```python
from build123d import *

# Parameters (mm, degrees)
SKETCH1_W           = 70
SKETCH1_H           = 70
BOSS_EXTRUDE1_DEPTH = 10
SKETCH2_R           = 30
SKETCH2_R_2         = 27.45
BOSS_EXTRUDE2_DEPTH = 5
FILLET1_R           = 2.5
BOSS_EXTRUDE3_DEPTH = 10
SKETCH5_R           = 1.5
SKETCH5_W           = 70
SKETCH5_H           = 10
BOSS_EXTRUDE5_DEPTH = 3


with BuildPart() as part:
    # Sketch1 → Boss-Extrude1 (new body)
    with BuildSketch(Plane.XY):
        Rectangle(SKETCH1_W, SKETCH1_H)
    extrude(amount=BOSS_EXTRUDE1_DEPTH)

    # Sketch2 → Boss-Extrude2 (add)
    with BuildSketch(Plane.XY.offset(10)):
        Circle(SKETCH2_R)
        Circle(SKETCH2_R_2, mode=Mode.SUBTRACT)
    extrude(amount=BOSS_EXTRUDE2_DEPTH)

    # Fillet1
    fillet1_edges = [part.edges().sort_by_distance(p)[0] for p in [
        (-35, 35, 5),
        (35, 35, 5),
    ]]
    fillet(fillet1_edges, radius=FILLET1_R)

    # Sketch3 → Boss-Extrude3 (add)
    with BuildSketch(Plane(origin=(0, 0, 0), x_dir=(-1, 0, 0), z_dir=(0, 0, -1))):
        Polygon((-20.75, -38.5), (-15.75, -38.5), (-15.75, -41.5), (-30.75, -41.5), (-30.75, -38.5), (-25.75, -38.5), (-25.75, -35), (-20.75, -35), align=None)
        Polygon((30.75, -38.5), (30.75, -41.5), (15.75, -41.5), (15.75, -38.5), (20.75, -38.5), (20.75, -35), (25.75, -35), (25.75, -38.5), align=None)
    extrude(amount=-BOSS_EXTRUDE3_DEPTH)

    # Sketch5 → Boss-Extrude5 (add)
    with BuildSketch(Plane.XZ.offset(35)):
        with BuildLine():
            Line((5, -5), (35, -5))
            ThreePointArc((35, -5), (38.535533906, -3.535533906), (40, 0))
            Line((40, 0), (40, 10))
            ThreePointArc((40, 10), (38.535533906, 13.535533906), (35, 15))
            Line((35, 15), (-35, 15))
            ThreePointArc((-35, 15), (-38.535533906, 13.535533906), (-40, 10))
            Line((-40, 10), (-40, 0))
            ThreePointArc((-40, 0), (-38.535533906, -3.535533906), (-35, -5))
            Line((-35, -5), (-5, -5))
            Line((-5, -5), (-5, -5.5))
            ThreePointArc((-5, -5.5), (-4.853553391, -5.853553391), (-4.5, -6))
            Line((-4.5, -6), (4.5, -6))
            ThreePointArc((4.5, -6), (4.853553391, -5.853553391), (5, -5.5))
            Line((5, -5.5), (5, -5))
        make_face()
        with Locations(Location((0, -3, 0), (0, 0, 270))):
            Circle(SKETCH5_R, mode=Mode.SUBTRACT)
        with Locations((0, 5)):
            Rectangle(SKETCH5_W, SKETCH5_H, mode=Mode.SUBTRACT)
    extrude(amount=-BOSS_EXTRUDE5_DEPTH)


solid = part.part
```
For this review, take the finished solid that the model builds, in its own axes (mm). A direction names the side the tool comes from. Round coordinates to 2 decimals unless told otherwise and drop trailing zeros. Write each loop counter-clockwise with the first axis right and the second up, starting at its lowest first coordinate (ties: lowest second). Pieces come first, ordered by that corner, then holes. Notation, with made-up numbers: (3.25, 75.5) -> (48.25, 75.5) arc R16 ccw to (48.25, 102.5) -> close; hole circle Ø5 at (-19, 75). An arc over 180 degrees is marked (long way). One line per question, with ' | ' between items. Start each with the question number.
(1) Mouldability with a two-part tool opening along Y and no side actions: class faces 4 (the face through (-40, -34, 5)), 5 (the face through (-29.97, 1.32, 12.46)), 6 (the face through (23, -41.5, 5)) as released by +Y, released by -Y, zero draft, split by the parting line, or undercut.
(2) Add section B-B, the plane x = 0. Write out the cut boundary in (y, z).
(3) Tool access review of faces 1 (the face through (23, -39, 10)), 2 (the face through (23, -39, 0)), 3 (the face through (-28, -38.5, 5)): name each direction out of +Z, -Z, +X, -X, +Y, -Y from which nothing blocks a thin tool from reaching the whole face with its end or side.
(4) Insertion check: P1, Ø6, axis at y = 24, z = 9.5, coming from the -X side; P2, Ø5, axis at x = -0.5, y = 20.5, coming from the -Z side; P3, Ø0.9, axis at y = -40.5, z = 6.5, coming from the +X side. Each pin has a flat end and moves straight along its axis. Give the tip position at first contact, or say it passes through.
(5) For line 1 along Y through (x, z) = (0, 13.25); line 2 along Y through (x, z) = (-30, 7.5); line 3 along X through (y, z) = (-35.5, 3.75), list the stretches that pass through material, from the lowest coordinate up. Write a range as from..to.
(6) Add section C-C, the plane y = 0. Write out the cut boundary in (x, z), plus the area to 4 significant figures.
(7) Add section A-A, the plane z = -3. Write out the cut boundary in (x, y).
(8) Add section D-D, the plane z = 2. Write out the cut boundary in (x, y).
Answer list:
1) face 4: zero draft | face 5: undercut | face 6: released by -Y
2) outline: (-35, -6) -> (-32, -6) -> (-32, -4.5) -> (-35, -4.5) -> close; (-35, -1.5) -> (-32, -1.5) -> (-32, 0) -> (35, 0) -> (35, 10) -> (30, 10) -> (30, 15) -> (27.45, 15) -> (27.45, 10) -> (-27.45, 10) -> (-27.45, 15) -> (-30, 15) -> (-30, 10) -> (-32, 10) -> (-32, 15) -> (-35, 15) -> close
3) face 1: +Z, +X, -X, -Y | face 2: -Z, +X, -X, -Y | face 3: +Z, -Z, -X
4) P1: x = -35 | P2: z = 0 | P3: x = 30.75
5) line 1: -35..-32, -30..-27.45, 27.45..30 | line 2: -41.5..-38.5, -35..35 | line 3: -25.75..-20.75, 20.75..25.75
6) outline: (-35, 0) -> (35, 0) -> (35, 10) -> (30, 10) -> (30, 15) -> (27.45, 15) -> (27.45, 10) -> (-27.45, 10) -> (-27.45, 15) -> (-30, 15) -> (-30, 10) -> (-35, 10) -> close | area: 725.5 mm²
7) outline: (-39, -35) -> (-1.5, -35) -> (-1.5, -32) -> (-39, -32) -> close; (1.5, -35) -> (39, -35) -> (39, -32) -> (1.5, -32) -> close
8) outline: (-40, -35) -> (-25.75, -35) -> (-25.75, -38.5) -> (-30.75, -38.5) -> (-30.75, -41.5) -> (-15.75, -41.5) -> (-15.75, -38.5) -> (-20.75, -38.5) -> (-20.75, -35) -> (20.75, -35) -> (20.75, -38.5) -> (15.75, -38.5) -> (15.75, -41.5) -> (30.75, -41.5) -> (30.75, -38.5) -> (25.75, -38.5) -> (25.75, -35) -> (40, -35) -> (40, -32) -> (35, -32) -> (35, 32.5) arc R2.5 ccw to (32.5, 35) -> (-32.5, 35) arc R2.5 ccw to (-35, 32.5) -> (-35, -32) -> (-40, -32) -> close
